from build123d import *

# Parameters (mm, degrees)
SKETCH1_W           = 85
SKETCH1_H           = 220
SKETCH1_W_2         = 70
SKETCH1_H_2         = 205
BOSS_EXTRUDE1_DEPTH = 7.5
SKETCH2_R           = 1.45
CUT_EXTRUDE1_DEPTH  = 10
CUT_EXTRUDE2_START  = -10
SKETCH3_R           = 1.45
CUT_EXTRUDE2_DEPTH  = 10
BOSS_EXTRUDE3_DEPTH = 85
BOSS_EXTRUDE4_DEPTH = 20
BOSS_EXTRUDE5_DEPTH = 20


with BuildPart() as part:
    # Sketch1 → Boss-Extrude1 (new body)
    with BuildSketch(Plane(origin=(0, 0, 0), x_dir=(0, 1, 0), z_dir=(0, 0, 1))):
        Rectangle(SKETCH1_W, SKETCH1_H)
        Rectangle(SKETCH1_W_2, SKETCH1_H_2, mode=Mode.SUBTRACT)
    extrude(amount=BOSS_EXTRUDE1_DEPTH)

    # Sketch2 → Cut-Extrude1 (cut)
    with BuildSketch(Plane(origin=(-110, 0, 0), x_dir=(0, -1, 0), z_dir=(-1, 0, 0))):
        with Locations(Location((-38.75, 3.75, 0), (0, 0, 90))):
            Circle(SKETCH2_R)
        with Locations(Location((38.75, 3.75, 0), (0, 0, 90))):
            Circle(SKETCH2_R)
    extrude(amount=-CUT_EXTRUDE1_DEPTH, mode=Mode.SUBTRACT)

    # Sketch3 → Cut-Extrude2 (cut)
    with BuildSketch(Plane.YZ.offset(110).offset(CUT_EXTRUDE2_START)):
        with Locations(Location((-38.75, 3.75, 0), (0, 0, 90))):
            Circle(SKETCH3_R)
        with Locations(Location((38.75, 3.75, 0), (0, 0, 90))):
            Circle(SKETCH3_R)
    extrude(amount=CUT_EXTRUDE2_DEPTH, mode=Mode.SUBTRACT)

    # Sketch5 → Boss-Extrude3 (add, through all)
    with BuildSketch(Plane(origin=(0, 42.5, 0), x_dir=(-1, 0, 0), z_dir=(0, 1, 0))):
        Polygon((-110, 7.5), (-110, 15), (-102.5, 7.5), align=None)
    extrude(amount=-BOSS_EXTRUDE3_DEPTH)

    # Sketch5<4> → Boss-Extrude4 (add)
    with BuildSketch(Plane(origin=(0, 42.5, 0), x_dir=(-1, 0, 0), z_dir=(0, 1, 0))):
        Polygon((110, 7.5), (110, 15), (102.5, 7.5), align=None)
    extrude(amount=-BOSS_EXTRUDE4_DEPTH)

    # Sketch4 → Boss-Extrude5 (add)
    with BuildSketch(Plane.XZ.offset(42.5)):
        Polygon((-110, 15), (-110, 7.5), (-102.5, 7.5), align=None)
    extrude(amount=-BOSS_EXTRUDE5_DEPTH)


solid = part.part
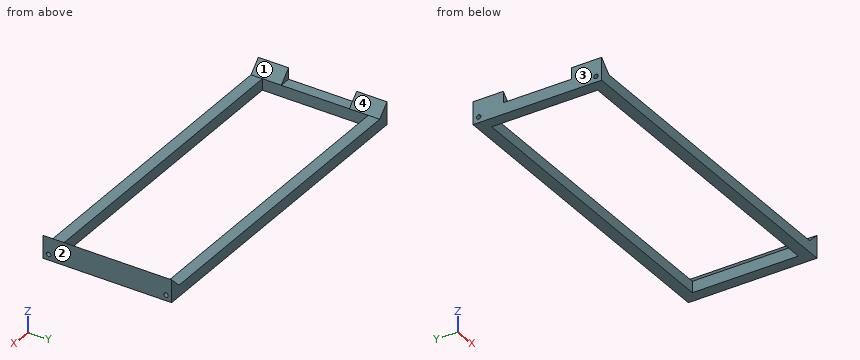
Here's how the part is built. I have some questions about the finished solid (model axes, mm). Face numbers are marked on the shaded views. Coordinates: 2 decimals unless noted, no trailing zeros. Loops run counter-clockwise (first coordinate to the right, second up) from the corner with the lowest first, then second, coordinate; pieces in that order, holes last.
1. Imagine slicing it at A-A, the plane y = -1. Please give me the cut outline in (x, z).
2. If we mould it in two halves opening along X, with no side actions, what happens to the marked faces 1, 2, 3 and 4? For each: pulls with the +X half, pulls with the -X half, needs draft (parallel to the pull), parting line crosses it, or undercut.
3. Imagine slicing it at B-B, the plane z = 11.25. Please give me the cut outline in (x, y).
4. For P1, Ø0.9, axis at y = 38.5, z = 3.5, coming from the -X side; P2, Ø1.5, axis at x = -87.5, z = 9, coming from the +Y side; P3, Ø1, axis at y = 9.5, z = 13, coming from the -X side; P4, Ø8, axis at x = -49.5, y = 38.5, coming from the +Z side, each with a flat end and sliding along its axis, tell me the tip position at first contact or that it passes through.
5. I need wall thicknesses on L1, parallel to Y at x = -107.25, z = 3.75; L2, parallel to X at y = 6, z = 6; L3, parallel to Y at x = -91, z = 2.5. Which ranges of each line are inside material? Lowest first, please.
6. Imagine slicing it at C-C, the plane x = -35. Please give me the cut outline in (y, z).
Taken from the geometry:
1. outline: (-110, 0) - (-102.5, 0) - (-102.5, 7.5) - (-110, 7.5) - close; (102.5, 0) - (110, 0) - (110, 15) - (102.5, 7.5) - close
2. face 1: undercut
2. face 2: pulls with the +X half
2. face 3: pulls with the -X half
2. face 4: undercut
3. outline: (-110, -42.5) - (-106.25, -42.5) - (-106.25, -22.5) - (-110, -22.5) - close; (-110, 22.5) - (-106.25, 22.5) - (-106.25, 42.5) - (-110, 42.5) - close; (106.25, -42.5) - (110, -42.5) - (110, 42.5) - (106.25, 42.5) - close
4. P1: stops at x = -100
4. P2: passes through
4. P3: stops at x = 107.5
4. P4: stops at z = 7.5
5. L1: y = -42.5 to -40.2, -37.3 to 37.3, 40.2 to 42.5
5. L2: x = -110 to -102.5, 102.5 to 110
5. L3: y = -42.5 to -35, 35 to 42.5
6. outline: (-42.5, 0) - (-35, 0) - (-35, 7.5) - (-42.5, 7.5) - close; (35, 0) - (42.5, 0) - (42.5, 7.5) - (35, 7.5) - close
